For this review, take the finished solid that the model builds, in its own axes (mm). Give positions to 0.01 mm unless a question says otherwise; leave off trailing zeros. Use CSV: the item, a comma, the result in double quotes. Start each with the question number.
1. Take a section at A-A, the plane x = -2.5. State how many separate pieces and enclosed holes the cut face has, and give its area (3 significant figures).
2. Insertion check: P1, Ø3.5, axis at y = 2.5, z = 9, coming from the -X side; P2, Ø6, axis at y = -157, z = 0, coming from the -X side; P3, Ø1.5, axis at x = -1.5, y = 6, coming from the +Z side; P4, Ø4.5, axis at y = 157, z = 0, coming from the -X side. Each pin has a flat end and moves straight along its axis. Give the tip position at first contact, or say it passes through.
3. To check wall thickness, follow line 1 (Y direction, x = -2.5, z = 0); line 2 (Y direction, x = -1.5, z = -6.5); line 3 (X direction, y = 23.7, z = -8). State the ranges of each line that lie inside material, in increasing order. Write a range as [from, to].
from build123d import *

# Parameters (mm, degrees)
SKETCH2_W               = 10
SKETCH2_H               = 23
BOSS_EXTRUDE1_DEPTH     = 175
SKETCH3_R               = 2.5
CUT_EXTRUDE1_DEPTH      = 176.662318099
SKETCH5_R               = 2.5
CUT_EXTRUDE2_DEPTH      = 176.662318099
SKETCH6_W               = 5
SKETCH6_H               = 40
CUT_EXTRUDE3_DEPTH      = 7
SKETCH7_R               = 1.5
CUT_EXTRUDE6_DEPTH      = 5
MIRROR2_COPY_1_SKETCH_R = 1.5
MIRROR2_COPY_1_DEPTH    = 5


with BuildPart() as part:
    # Sketch2 → Boss-Extrude1 (new, symmetric)
    with BuildSketch(Plane(origin=(0, 0, 0), x_dir=(1, 0, 0), z_dir=(0, 1, 0))):
        Rectangle(SKETCH2_W, SKETCH2_H)
    extrude(amount=BOSS_EXTRUDE1_DEPTH, both=True)

    # Sketch3 → Cut-Extrude1 (cut, through all)
    with BuildSketch(Plane(origin=(5, 0, 0), x_dir=(0, 0, -1), z_dir=(1, 0, 0))):
        with Locations((0, 167)):
            Circle(SKETCH3_R)
        with Locations((0, 157)):
            Circle(SKETCH3_R)
    extrude(amount=-CUT_EXTRUDE1_DEPTH, mode=Mode.SUBTRACT)

    # Sketch5 → Cut-Extrude2 (cut, through all)
    with BuildSketch(Plane(origin=(5, 0, 0), x_dir=(0, 0, -1), z_dir=(1, 0, 0))):
        with Locations((0, -167)):
            Circle(SKETCH5_R)
        with Locations((0, -157)):
            Circle(SKETCH5_R)
    extrude(amount=-CUT_EXTRUDE2_DEPTH, mode=Mode.SUBTRACT)

    # Sketch6 → Cut-Extrude3 (cut)
    with BuildSketch(Plane.XY.offset(11.5)):
        with Locations((-2.5, 0)):
            Rectangle(SKETCH6_W, SKETCH6_H)
    cut_extrude3 = extrude(amount=-CUT_EXTRUDE3_DEPTH, mode=Mode.SUBTRACT)

    # Sketch7 → Cut-Extrude6 (cut)
    with BuildSketch(Plane.XZ.offset(-20)):
        with Locations(Location((-2.5, 8, 0), (0, 0, 270))):
            Circle(SKETCH7_R)
    cut_extrude6 = extrude(amount=-CUT_EXTRUDE6_DEPTH, mode=Mode.SUBTRACT)

    # Mirror1: Cut-Extrude6 across plane
    add(cut_extrude6.mirror(Plane(origin=(0, 0, 0), x_dir=(0, 0, 1), z_dir=(0, -1, 0))), mode=Mode.SUBTRACT)

    # Mirror2: Cut-Extrude3, Cut-Extrude6 across plane
    add(cut_extrude3.mirror(Plane.XY), mode=Mode.SUBTRACT)
    add(cut_extrude6.mirror(Plane.XY), mode=Mode.SUBTRACT)

    # Mirror2 copy 1 sketch → Mirror2 copy 1 (cut)
    with BuildSketch(Plane(origin=(0, -20, 0), x_dir=(1, 0, 0), z_dir=(0, 1, 0))):
        with Locations(Location((-2.5, 8, 0), (0, 0, 270))):
            Circle(MIRROR2_COPY_1_SKETCH_R)
    extrude(amount=-MIRROR2_COPY_1_DEPTH, mode=Mode.SUBTRACT)


solid = part.part
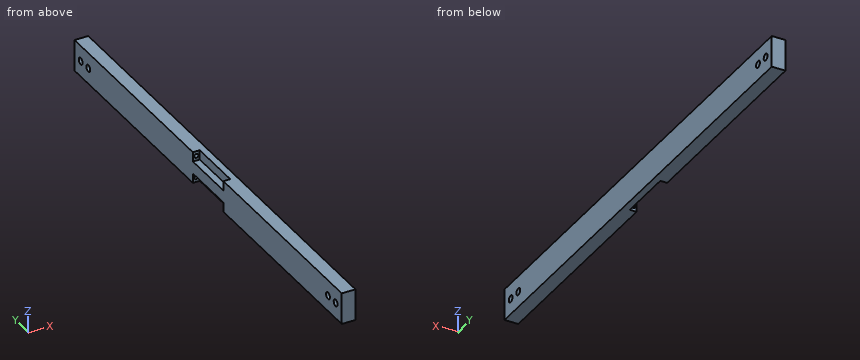
Result set:
1,separate pieces,"1"
1,enclosed holes,"4"
1,area,"7,350 mm2"
2,P1,"x = 0"
2,P2,"x = -5"
2,P3,"z = 4.5"
2,P4,"through"
3,line 1,"[-175, -169.5], [-164.5, -159.5], [-154.5, 154.5], [159.5, 164.5], [169.5, 175]"
3,line 2,"[-175, -20], [20, 175]"
3,line 3,"[-5, -4], [-1, 5]"
